Autodesk Inventor part; units mm, degrees
ref_plane "YZ Plane" through (0, 0, 0) normal (1, 0, 0) x (0, 1, 0)
ref_plane "XZ Plane" through (0, 0, 0) normal (0, 1, 0) x (-1, 0, 0)
ref_plane "XY Plane" through (0, 0, 0) normal (0, 0, 1) x (1, 0, 0)
sketch "Sketch1" plane through (0, 0, 0) normal (0, 0, 1) x (1, 0, 0)
  line L0 (0, 0) -> (0, 88.9)
  line L1 (0, 88.9) -> (25.4, 88.9)
  line L2 (25.4, 88.9) -> (25.4, 57.9416)
  line L3 (25.4, 57.9416) -> (72.9934, 19.8257)
  line L4 (72.9934, 19.8257) -> (57.1157, 0)
  line L5 (57.1157, 0) -> (25.4, 25.4)
  line L6 (25.4, 25.4) -> (25.4, 0)
  line L7 (25.4, 0) -> (0, 0)
  dimension "d0" = 25.4
  dimension "d1" = 25.4
  dimension "d3" = 25.4
  dimension "d5" = 51.31
  dimension "d18" = 88.9
extrude "Extrusion1" add sketch "Sketch1" along normal blind 2.032
sketch "Sketch3" plane through (0, 0, 2.032) normal (0, 0, 1) x (1, 0, 0)
  line L0 (25.4, 57.9416) -> (25.4, 88.9)
  line L1 (0, 0) -> (25.4, 0)
  line L2 (72.9934, 19.8257) -> (25.4, 57.9416)
  line L3 (57.1157, 0) -> (72.9934, 19.8257)
  point P0 (12.7, 12.7)
  point P1 (12.7, 25.4)
  point P2 (12.7, 38.1)
  point P3 (12.7, 50.8)
  point P4 (12.7, 63.5)
  point P5 (12.7, 76.2)
  point P6 (55.1417, 17.8517)
  point P7 (45.2289, 25.7906)
  point P8 (35.316, 33.7294)
  dimension "d8" = 12.7
  dimension "d9" = 12.7
  dimension "d10" = 12.7
  dimension "d11" = 12.7
  dimension "d12" = 12.7
  dimension "d13" = 12.7
  dimension "d14" = 12.7
  dimension "d19" = 12.7
  dimension "d20" = 12.7
  dimension "d21" = 12.7
  dimension "d23" = 12.7
  dimension "d24" = 12.7
  dimension "d25" = 12.7
hole "Hole1" at (12.7, 12.7, 2.032) at (12.7, 25.4, 2.032) at (12.7, 38.1, 2.032) at (12.7, 50.8, 2.032) at (12.7, 63.5, 2.032) at (12.7, 76.2, 2.032) at (55.1417, 17.8517, 2.032) at (45.2289, 25.7906, 2.032) at (35.316, 33.7294, 2.032) direction (0, 0, -1) diameter 4.8514 end through all
properties part number "SUP_011_Top4BarBarGusset" material "Aluminum 6061"
CAD build for the part. Positions are in the model's coordinates, mm. A direction names the side the tool comes from. Coordinates: 2 decimals unless noted, no trailing zeros. Write each loop counter-clockwise with the first axis right and the second up, starting at its lowest first coordinate (ties: lowest second). Pieces come first, ordered by that corner, then holes. Notation, with made-up numbers: M -30.5,21.5 L -9.5,21.5 A18 ccw -9.5,25.5 Z; hole C -35.75,50 d11. An arc over 180 degrees is marked long. Answer as a JSON object with one key per item and string values. Group by question number.
1) Saw through at D-D (y = 12.7). Write the cut outline in (x, z), plus the area to 3 significant figures.
2) Wall check: line 1 (X direction, y = 76.2, z = 1.05); line 2 (X direction, y = 16, z = 1.9); line 3 (X direction, y = 12.7, z = 0.8). Give the ranges that are in metal, low to high. Write a range as from..to.
3) Pin check, flat tips, straight feed: pin 1 Ø1 at (x, y) = (27.5, 63.5) entering from -Z; pin 2 Ø8 at (x, y) = (12.7, 25.4) entering from +Z. Stop position of each tip, or through.
4) Saw through at B-B (y = 63.5). Write the cut outline in (x, z).
5) Tool access for faces 4 (the face through (25.4, 74, 1)), 5 (the face through (25.4, 13, 1)), 6 (the face through (13.63, 23.16, 1)): list every direction of +Z, -Z, +X, -X, +Y, -Y with a clear straight run to the whole face (end or side of a thin tool).
6) Saw through at C-C (z = 0.9). Give the number of separate pieces and of enclosed holes in the cut face, plus the area to 3 significant figures.
7) Mould opens along Y. For faces 1 (the face through (37.684, 34.255, 1.002)), 2 (the face through (28, 35, 0)), 3 (the face through (65.166, 10.052, 1.002)) say: +Y half, -Y half, draft (parallel to the pull), parting line (faces both ways), or undercut.
8) Saw through at A-A (x = 12.7). Write the cut outline in (y, z), plus the area to 3 significant figures.
Values follow:
{
 "1": {"outline": "M 0,0 L 10.27,0 L 10.27,2.03 L 0,2.03 Z; M 15.13,0 L 25.4,0 L 25.4,2.03 L 15.13,2.03 Z; M 41.26,0 L 67.29,0 L 67.29,2.03 L 41.26,2.03 Z", "area": "94.6 mm2"},
 "2": {"line 1": "x = 0..10.27, 15.13..25.4", "line 2": "x = 0..25.4, 37.14..53.57, 56.71..69.93", "line 3": "x = 0..10.27, 15.13..25.4, 41.26..67.29"},
 "3": {"pin 1": "passes through", "pin 2": "stops at z = 2.03"},
 "4": {"outline": "M 0,0 L 10.27,0 L 10.27,2.03 L 0,2.03 Z; M 15.13,0 L 25.4,0 L 25.4,2.03 L 15.13,2.03 Z"},
 "5": {"face 4": "+Z, -Z, +X, +Y", "face 5": "+Z, -Z, -Y", "face 6": "+Z, -Z"},
 "6": {"separate pieces": "1", "enclosed holes": "9", "area": "3,380 mm2"},
 "7": {"face 1": "undercut", "face 2": "draft", "face 3": "-Y half"},
 "8": {"outline": "M 0,0 L 10.27,0 L 10.27,2.03 L 0,2.03 Z; M 15.13,0 L 22.97,0 L 22.97,2.03 L 15.13,2.03 Z; M 27.83,0 L 35.67,0 L 35.67,2.03 L 27.83,2.03 Z; M 40.53,0 L 48.37,0 L 48.37,2.03 L 40.53,2.03 Z; M 53.23,0 L 61.07,0 L 61.07,2.03 L 53.23,2.03 Z; M 65.93,0 L 73.77,0 L 73.77,2.03 L 65.93,2.03 Z; M 78.63,0 L 88.9,0 L 88.9,2.03 L 78.63,2.03 Z", "area": "121 mm2"}
}
